Can you work these out from the model? Positions are in its coordinate system, mm. A direction names the side the tool comes from. Round coordinates to 2 decimals unless told otherwise and drop trailing zeros. Loops run counter-clockwise (first coordinate to the right, second up) from the corner with the lowest first, then second, coordinate; pieces in that order, holes last.
(1) If I drill on line 1 along X through (y, z) = (54, 6.75); line 2 along Y through (x, z) = (69.5, 13.25); line 3 along X through (y, z) = (-15, 6), over which ranges is the centre line in solid material (lowest first)?
(2) I want a section at B-B on y = 31. Write out the boundary of the cut face in (x, z).
(3) Which directions (+Z, -Z, +X, -X, +Y, -Y) give clear straight access to the entire face, cutting with the end or side of a thin tool? Please do faces 4 (the face through (56, 20, 12)), 5 (the face through (44, 40, 12)), 6 (the face through (-1, 1, 25)), 7 (the face through (38.81, 52.97, 12.32)), 8 (the face through (-44, 40, 12)).
(4) Thinking about a two-plate mould opening in X: for faces 1 (the face through (-1, -60, 12)), 2 (the face through (-41, -25, 12)), 3 (the face through (-39.944, 57.723, 12.325)), which applies, released by +X, released by -X, zero draft, split by the parting line, or undercut?
(5) I want a section at C-C on z = 20. Give the number of separate pieces and of enclosed holes in the cut face, plus the area to 3 significant figures.
(6) Will these pins go through, and if not, where does the flat tip stop? pin 1 Ø12.5 at (x, z) = (63, 15.5) entering from -Y; pin 2 Ø7.5 at (x, z) = (-54, 17.5) entering from +Y; pin 3 Ø6 at (y, z) = (-38.5, 4.5) entering from -X.
(7) I want a section at A-A on x = -60. Write out the boundary of the cut face in (y, z), plus the area to 3 significant figures.
from build123d import *

# Parameters (mm, degrees)
F0_W     = 40
F0_H     = 40
F0_R     = 1.5
F1_DEPTH = 25


with BuildPart() as f1:
    # F0 (on Top) → F1 (new body)
    with BuildSketch(Plane.XY):
        with Locations((-56, 0)):
            Rectangle(F0_W, F0_H)
        with Locations((-69.8812, -16)):
            Circle(F0_R, mode=Mode.SUBTRACT)
        with Locations((-42.1188, -16)):
            Circle(F0_R, mode=Mode.SUBTRACT)
        with Locations((-69.8812, 16)):
            Circle(F0_R, mode=Mode.SUBTRACT)
        with Locations((-42.1188, 16)):
            Circle(F0_R, mode=Mode.SUBTRACT)
        Polygon((0, 20), (-36, 20), (-36, -20), (0, -20), (36, -20), (36, 20), align=None)
        Polygon((0, -20), (-36, -20), (-36, -60), (0, -60), (36, -60), (36, -20), align=None)
        Polygon((-36, -60), (-36, -20), (-44, -24.618802), (-44, -55.381198), align=None)
        with Locations((-40, -53.881198)):
            Circle(F0_R, mode=Mode.SUBTRACT)
        with Locations((-40, -26.118802)):
            Circle(F0_R, mode=Mode.SUBTRACT)
        Polygon((44, -24.618802), (36, -20), (36, -60), (44, -55.381198), align=None)
        with Locations((40, -53.881198)):
            Circle(F0_R, mode=Mode.SUBTRACT)
        with Locations((40, -26.118802)):
            Circle(F0_R, mode=Mode.SUBTRACT)
        Polygon((-36, 60), (-36, 20), (0, 20), (36, 20), (36, 60), (0, 60), align=None)
        with Locations((-34.410123, 56.457806)):
            Circle(F0_R, mode=Mode.SUBTRACT)
        Polygon((-44, 24.618802), (-36, 20), (-36, 60), (-44, 55.381198), align=None)
        with Locations((-40, 26.118802)):
            Circle(F0_R, mode=Mode.SUBTRACT)
        with Locations((-40, 53.881198)):
            Circle(F0_R, mode=Mode.SUBTRACT)
        with Locations((56, 0)):
            Rectangle(F0_W, F0_H)
        with Locations((42.1188, -16)):
            Circle(F0_R, mode=Mode.SUBTRACT)
        with Locations((69.8812, -16)):
            Circle(F0_R, mode=Mode.SUBTRACT)
        with Locations((42.1188, 16)):
            Circle(F0_R, mode=Mode.SUBTRACT)
        with Locations((69.8812, 16)):
            Circle(F0_R, mode=Mode.SUBTRACT)
        Polygon((36, 60), (36, 20), (44, 24.618802), (44, 55.381198), align=None)
        with Locations((40, 26.118802)):
            Circle(F0_R, mode=Mode.SUBTRACT)
        with Locations((40, 53.881198)):
            Circle(F0_R, mode=Mode.SUBTRACT)
    extrude(amount=F1_DEPTH)


solid = f1.part
Filled sheet:
1. line 1: x = -44 to -41.5, -38.5 to 38.5, 41.5 to 44
1. line 2: y = -20 to -17.45, -14.55 to 14.55, 17.45 to 20
1. line 3: x = -76 to -71, -68.76 to -43.24, -41 to 41, 43.24 to 68.76, 71 to 76
2. outline: (-44, 0) - (44, 0) - (44, 25) - (-44, 25) - close
3. face 4: +Z, -Z, +X
3. face 5: +Z, -Z, +X, +Y
3. face 6: +Z, +X, -X, +Y, -Y
3. face 7: +Z, -Z
3. face 8: +Z, -Z, -X, +Y
4. face 1: zero draft
4. face 2: undercut
4. face 3: released by -X
5. separate pieces: 1
5. enclosed holes: 17
5. area: 12,900 mm2
6. pin 1: stops at y = -20
6. pin 2: stops at y = 20
6. pin 3: stops at x = -44
7. outline: (-20, 0) - (20, 0) - (20, 25) - (-20, 25) - close
7. area: 1,000 mm2
